```python
from build123d import *

# Parameters (mm, degrees)
F0_W           = 220
F0_H           = 110
F1_DEPTH       = 10
F2_R           = 5
F2_R_2         = 2
F3_DEPTH       = 10.001
F4_D           = 3.3
F5_D           = 5
F5_CBORE_D     = 8.25
F5_CBORE_DEPTH = 4
F6_SIZE        = 1


with BuildPart() as f1:
    # F0 (on Top) → F1 (new body)
    with BuildSketch(Plane.XY):
        Rectangle(F0_W, F0_H)
    extrude(amount=F1_DEPTH)

    # F2 (on face) → F3 (cut, through all)
    with BuildSketch(Plane(origin=(0, 0, 0), x_dir=(1, 0, 0), z_dir=(0, 0, -1))):
        with Locations((50, 30)):
            Circle(F2_R)
        with Locations((-20, -45)):
            Circle(F2_R_2)
        with Locations((10, -45)):
            Circle(F2_R_2)
    extrude(amount=-F3_DEPTH, mode=Mode.SUBTRACT)

    # F4 (through all)
    with Locations(Plane(origin=(0, 0, 0), x_dir=(1, 0, 0), z_dir=(0, 0, -1))):
        with Locations((95, -5), (95, 15)):
            Hole(F4_D / 2)

    # F5 (through all)
    with Locations(Plane(origin=(0, 0, 0), x_dir=(1, 0, 0), z_dir=(0, 0, -1))):
        with Locations((-40, -45), (30, -45)):
            CounterBoreHole(F5_D / 2, F5_CBORE_D / 2, F5_CBORE_DEPTH)

    # F6
    f6_edges = [f1.edges().sort_by_distance(p)[0] for p in [
        (45, -30, 10),
    ]]
    chamfer(f6_edges, length=F6_SIZE)


solid = f1.part
```
Could you check a few things on this model? Use its own coordinates, in mm. A direction names the side the tool comes from. Round coordinates to 2 decimals unless told otherwise and drop trailing zeros. Loops run counter-clockwise (first coordinate to the right, second up) from the corner with the lowest first, then second, coordinate; pieces in that order, holes last.
Q1. I want a section at A-A (y = -30). Write out the boundary of the cut face in (x, z).
Q2. Please list where these lines run through material, in increasing order: L1, parallel to X at y = 45, z = 1.55 (3 decimals); L2, parallel to X at y = 45, z = 8.05; L3, parallel to Y at x = -20, z = 3.25.
Q3. I want a section at B-B (x = 30). Write out the boundary of the cut face in (y, z) (3 decimals).
Q4. On a 3-axis mill with a long thin cutter (end or side, diameter ignored), from which of +Z, -Z, +X, -X, +Y, -Y can I reach the whole of each face in a straight line? I mean faces 1 (the cylindrical face through (46, -27, 4)), 2 (the cylindrical face through (29, 49, 2)). Say none if no direction works.
Q5. For P1, Ø4, axis at x = 28.5, y = 45.5, coming from the -Z side, with a flat end and sliding along its axis, tell me the tip position at first contact or that it passes through.
Q6. Thinking about a two-plate mould opening in Y: for faces 3 (the flat face through (-2, 55, 5)), 4 (the flat face through (-2, 1, 10)), 5 (the cylindrical face through (-41, 49, 2)), 6 (the cylindrical face through (-42.31, 45.96, 7.04)), which applies, pulls with the +Y half, pulls with the -Y half, needs draft (parallel to the pull), parting line crosses it, or undercut?
Answer below:
1. outline: (-110, 0) - (45, 0) - (45, 9) - (44, 10) - (-110, 10) - close; (55, 0) - (110, 0) - (110, 10) - (56, 10) - (55, 9) - close
2. L1: x = -110 to -44.125, -35.875 to -22, -18 to 8, 12 to 25.875, 34.125 to 110
2. L2: x = -110 to -42.5, -37.5 to -22, -18 to 8, 12 to 27.5, 32.5 to 110
2. L3: y = -55 to 43, 47 to 55
3. outline: (-55, 0) - (40.875, 0) - (40.875, 4) - (42.5, 4) - (42.5, 10) - (-55, 10) - close; (47.5, 4) - (49.125, 4) - (49.125, 0) - (55, 0) - (55, 10) - (47.5, 10) - close
4. face 1: +Z, -Z
4. face 2: -Z
5. P1: stops at z = 4
6. face 3: pulls with the +Y half
6. face 4: needs draft
6. face 5: undercut
6. face 6: undercut
